```python
from build123d import *

# Parameters (mm, degrees)
BOSS_EXTRUDE1_DEPTH = 12
SKETCH2_R           = 25
BOSS_EXTRUDE2_DEPTH = 20
BOSS_EXTRUDE3_DEPTH = 4
SKETCH4_W           = 55
SKETCH4_H           = 12
CUT_EXTRUDE1_DEPTH  = 6
SKETCH5_R           = 10
CUT_EXTRUDE2_DEPTH  = 17
SKETCH6_W           = 125
SKETCH6_H           = 20
CUT_EXTRUDE3_DEPTH  = 6


with BuildPart() as part:
    # Sketch1 → Boss-Extrude1 (new body)
    with BuildSketch(Plane(origin=(0, 0, 0), x_dir=(1, 0, 0), z_dir=(0, 1, 0))):
        with BuildLine():
            Line((-30, 25), (30, 25))
            ThreePointArc((30, 25), (55, 0), (30, -25))
            Line((30, -25), (-30, -25))
            ThreePointArc((-30, -25), (-55, 0), (-30, 25))
        make_face()
    extrude(amount=BOSS_EXTRUDE1_DEPTH)

    # Sketch2 → Boss-Extrude2 (add)
    with BuildSketch(Plane(origin=(0, 12, 0), x_dir=(1, 0, 0), z_dir=(0, 1, 0))):
        with Locations(Location((-30, 0, 0), (0, 0, 270))):
            Circle(SKETCH2_R)
    extrude(amount=BOSS_EXTRUDE2_DEPTH)

    # Sketch3 → Boss-Extrude3 (add)
    with BuildSketch(Plane(origin=(0, 12, 0), x_dir=(1, 0, 0), z_dir=(0, 1, 0))):
        with BuildLine():
            Line((30, -12), (15, -12))
            ThreePointArc((15, -12), (3, 0), (15, 12))
            Line((15, 12), (30, 12))
            ThreePointArc((30, 12), (42, 0), (30, -12))
        make_face()
        with BuildLine():
            Line((30, -6), (15, -6))
            ThreePointArc((15, -6), (9, 0), (15, 6))
            Line((15, 6), (30, 6))
            ThreePointArc((30, 6), (36, 0), (30, -6))
        make_face(mode=Mode.SUBTRACT)
    extrude(amount=BOSS_EXTRUDE3_DEPTH)

    # Sketch4 → Cut-Extrude1 (cut)
    with BuildSketch(Plane(origin=(0, 32, 0), x_dir=(1, 0, 0), z_dir=(0, 1, 0))):
        with Locations((-30, 0)):
            Rectangle(SKETCH4_W, SKETCH4_H)
    extrude(amount=-CUT_EXTRUDE1_DEPTH, mode=Mode.SUBTRACT)

    # Sketch5 → Cut-Extrude2 (cut)
    with BuildSketch(Plane(origin=(0, 26, 0), x_dir=(1, 0, 0), z_dir=(0, 1, 0))):
        with Locations((-30, 0)):
            Circle(SKETCH5_R)
    extrude(amount=CUT_EXTRUDE2_DEPTH, mode=Mode.SUBTRACT)

    # Sketch6 → Cut-Extrude3 (cut)
    with BuildSketch(Plane.XZ):
        Rectangle(SKETCH6_W, SKETCH6_H)
    extrude(amount=-CUT_EXTRUDE3_DEPTH, mode=Mode.SUBTRACT)


solid = part.part
```
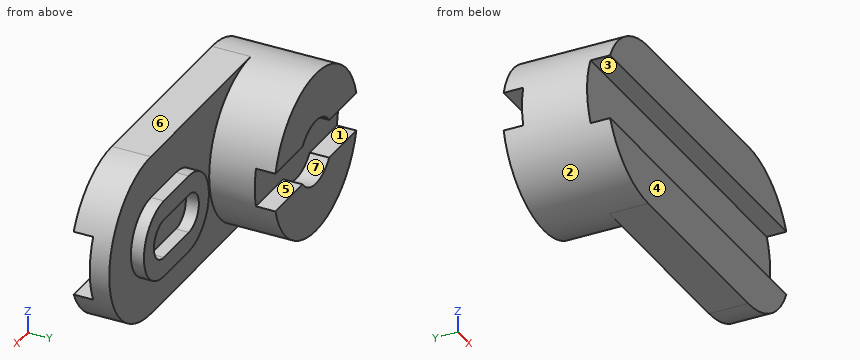
Work out the finished part from the listing and answer in its coordinate system (mm). Face numbers are marked on the shaded views. A direction names the side the tool comes from. Give positions to 0.01 mm unless a question says otherwise; leave off trailing zeros. Loops run counter-clockwise (first coordinate to the right, second up) from the corner with the lowest first, then second, coordinate; pieces in that order, holes last. Notation, with made-up numbers: M -2,79 L 26,79 A16 cw 26,88 Z; hole C 53,-11 d5. An arc over 180 degrees is marked long. One line per item, written item: value. Start each with the question number.
1. Determine the mould class of the marked faces 4, 5, 6 and 7 for opening direction Z: released by +Z, released by -Z, zero draft, split by the parting line, or undercut.
2. Find section D-D (z = -11). Give the vertices of the cut face in (x, y).
3. Each of these flat-tipped pins is pushed along its axis until it touches: P1, Ø3, axis at x = -49, y = 29.5, coming from the -Z side; P2, Ø3, axis at x = 43, y = 6, coming from the +Z side; P3, Ø3, axis at x = -44, y = 30, coming from the +Z side. Where does it stop, or does it pass through?
4. Find section C-C (y = 23). Give the vertices of the cut face in (x, z), and give its area (3 significant figures).
5. Find section A-A (z = 0). Give the vertices of the cut face in (x, y), and give its area (3 significant figures).
6. Find section B-B (x = 33). Give the vertices of the cut face in (y, z).
7. Which of the six approach directions +Z, -Z, +X, -X, +Y, -Y give full straight-line access (tool end or side, diameter ignored) to the marked faces 1, 2 and 3?
8. Find the intervals of material crossed by probe 1 along Z at (x, y) = (0.5, 2); probe 2 along X at (y, z) = (13, -0.5) (3 decimals); probe 3 along X at (y, z) = (13.5, 1), in increasing order.
Reported:
1. face 4: zero draft
1. face 5: undercut
1. face 6: released by +Z
1. face 7: undercut
2. outline: M -52.45,0 L 52.45,0 L 52.45,12 L 34.8,12 L 34.8,16 L 10.2,16 L 10.2,12 L -7.55,12 L -7.55,32 L -52.45,32 Z
3. P1: stops at z = -17.85
3. P2: stops at z = 22.2
3. P3: stops at z = 21.65
4. outline: C -30,0 d50
4. area: 1,960 mm²
5. outline: M -55,6 L 55,6 L 55,12 L 42,12 L 42,16 L 36,16 L 36,12 L 9,12 L 9,16 L 3,16 L 3,12 L -5,12 L -5,26 L -55,26 Z
5. area: 1,410 mm²
6. outline: M 0,-24.82 L 12,-24.82 L 12,-11.62 L 16,-11.62 L 16,-5.2 L 12,-5.2 L 12,5.2 L 16,5.2 L 16,11.62 L 12,11.62 L 12,24.82 L 0,24.82 L 0,10 L 6,10 L 6,-10 L 0,-10 Z
7. face 1: +X, -X, +Y
7. face 2: +Y
7. face 3: +X, -X, -Y
8. probe 1: z = -25 to -10, 10 to 25
8. probe 2: x = -54.995 to -5.005, 3.01 to 9.021, 35.979 to 41.99
8. probe 3: x = -54.98 to -5.02, 3.04 to 9.08, 35.92 to 41.96
